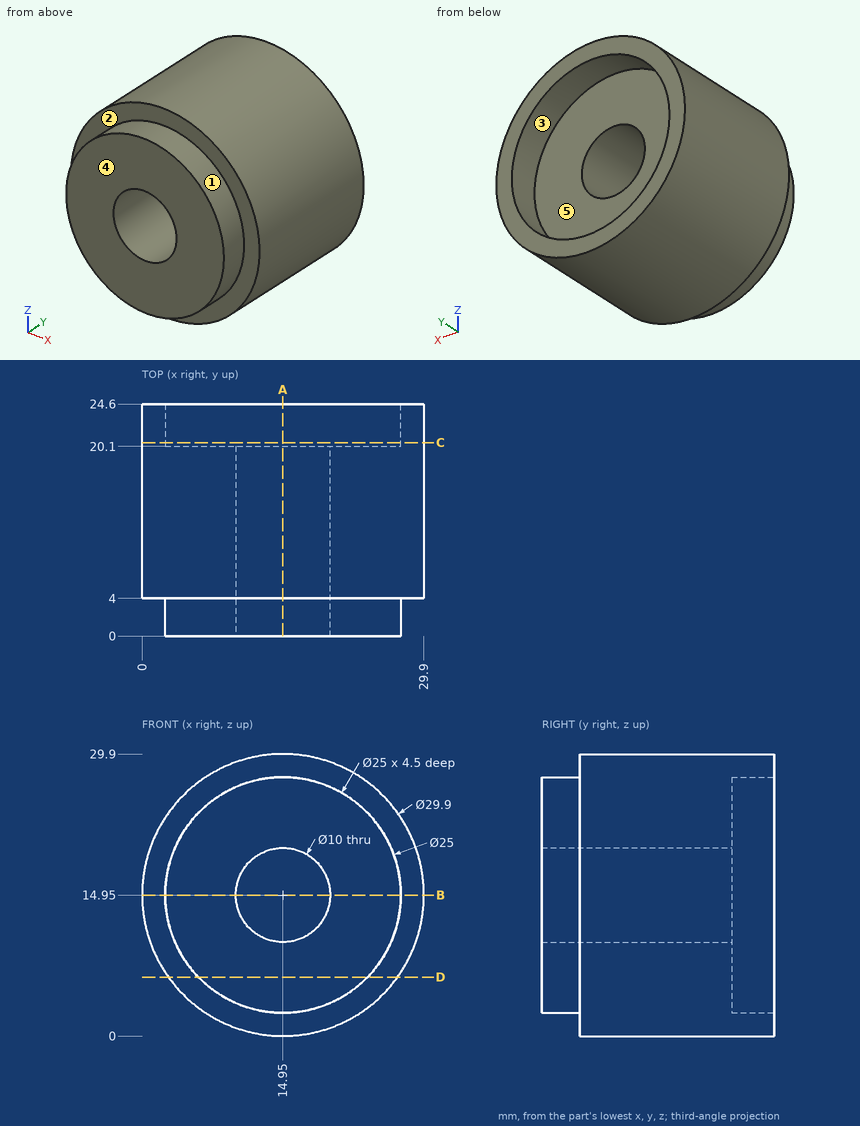
Part print with two shaded views. Sizes in mm from the minimum x, y, z corner. A direction names the side the tool comes from. Round coordinates to 2 decimals unless told otherwise and drop trailing zeros. Order: outer loops, then holes, each group sorted by start corner. A loop starts at its lowest first (then second) coordinate and runs counter-clockwise, first axis right, second up. Notation, with made-up numbers: M -9,-25 L 32,-25 A14 cw 32,2 Z; hole C -22.5,-32.5 d9. An arc over 180 degrees is marked long. Put each result on its own line as item: value. Start each with the question number.
1. Slice it at D-D on z = 6.25. List the corners of the cut face in (x, y).
2. Slice it at C-C on y = 20.5. List the corners of the cut face in (x, z), then the cut area to 3 significant figures.
3. Tool access for the marked faces 4 and 5: list every direction of +Z, -Z, +X, -X, +Y, -Y with a clear straight run to the whole face (end or side of a thin tool).
4. Drill centre lines: probe 1 along Z at (x, y) = (14.95, 13); probe 2 along X at (y, z) = (13.5, 15.25); probe 3 along Z at (x, y) = (14.95, 22.55). Where is each one in solid material? Low to high. Write a range as [from, to].
5. Slice it at A-A on x = 14.95. List the corners of the cut face in (y, z).
6. Two-plate mould, pull along Z, no slides. Class the marked faces 1, 2 and 3: +Z half, -Z half, draft (parallel to the pull), parting line (faces both ways), or undercut.
7. Slice it at B-B on z = 14.95. List the corners of the cut face in (x, y).
8. Drop flat-ended pins along their axis: pin 1 (12 mm diameter, centred on x = 25, y = 3.5, fed in from +Z); pin 2 (10 mm diameter, centred on x = 5.5, y = 14.5, fed in from +Z); pin 3 (1 mm diameter, centred on x = 24.5, y = 5.5, fed in from +Z); pin 4 (6 mm diameter, centred on x = 14.95, z = 14.95, fed in from -Y). Give the stop position or say it passes through.
Findings:
1. outline: M 2.79,4 L 5.97,4 L 5.97,0 L 23.93,0 L 23.93,4 L 27.11,4 L 27.11,24.6 L 23.93,24.6 L 23.93,20.1 L 5.97,20.1 L 5.97,24.6 L 2.79,24.6 Z
2. outline: C 14.95,14.95 d29.9; hole C 14.95,14.95 d25
2. area: 211 mm2
3. face 4: +Z, -Z, +X, -X, -Y
3. face 5: +Y
4. probe 1: [0, 9.95], [19.95, 29.9]
4. probe 2: [0, 9.96], [19.94, 29.9]
4. probe 3: [0, 2.45], [27.45, 29.9]
5. outline: M 0,2.45 L 4,2.45 L 4,0 L 24.6,0 L 24.6,2.45 L 20.1,2.45 L 20.1,9.95 L 0,9.95 Z; M 0,19.95 L 20.1,19.95 L 20.1,27.45 L 24.6,27.45 L 24.6,29.9 L 4,29.9 L 4,27.45 L 0,27.45 Z
6. face 1: parting line
6. face 2: draft
6. face 3: undercut
7. outline: M 0,4 L 2.45,4 L 2.45,0 L 9.95,0 L 9.95,20.1 L 2.45,20.1 L 2.45,24.6 L 0,24.6 Z; M 19.95,0 L 27.45,0 L 27.45,4 L 29.9,4 L 29.9,24.6 L 27.45,24.6 L 27.45,20.1 L 19.95,20.1 Z
8. pin 1: z = 29.34
8. pin 2: z = 29.22
8. pin 3: z = 26.85
8. pin 4: through
